```python
from build123d import *

# Parameters (mm, degrees)
F1_DEPTH = 15
F2_R     = 7.5
F3_DEPTH = 105.450168252
F4_R     = 10
F5_DEPTH = 70


with BuildPart() as f1:
    # F0 (on Front) → F1 (new body, symmetric)
    with BuildSketch(Plane.XZ):
        with BuildLine():
            Line((-21.2132034356, -21.2132034356), (-70.7106781187, -70.7106781187))
            ThreePointArc((-70.7106781187, -70.7106781187), (-38.2683432365, -92.3879532511), (0, -100))
            Line((0, -100), (0, -30))
            ThreePointArc((0, -30), (-11.480502971, -27.7163859753), (-21.2132034356, -21.2132034356))
        make_face()
        with BuildLine():
            Line((0, -30), (0, -100))
            ThreePointArc((0, -100), (38.2683432365, -92.3879532511), (70.7106781187, -70.7106781187))
            Line((70.7106781187, -70.7106781187), (21.2132034356, -21.2132034356))
            ThreePointArc((21.2132034356, -21.2132034356), (11.480502971, -27.7163859753), (0, -30))
        make_face()
    extrude(amount=F1_DEPTH, both=True)

    # F2 (on Top) → F3 (cut)
    with BuildSketch(Plane.XY):
        Circle(F2_R)
    extrude(amount=-F3_DEPTH, mode=Mode.SUBTRACT)

    # F4 (on Top) → F5 (cut)
    with BuildSketch(Plane.XY):
        Circle(F4_R)
    extrude(amount=-F5_DEPTH, mode=Mode.SUBTRACT)


solid = f1.part
```
Geometry: final body of the model. Coordinates: model frame, mm. A direction names the side the tool comes from. Coordinates: 2 decimals unless noted, no trailing zeros. Order: outer loops, then holes, each group sorted by start corner. A loop starts at its lowest first (then second) coordinate and runs counter-clockwise, first axis right, second up.
Item 1: Draft query along Y for faces 1 (the face through (46, 0, -46)), 2 (the face through (-1, 15, -60)), 3 (the face through (-7.493, 0.33, -84.79)). Return one class per face: released by +Y, released by -Y, zero draft, split by the parting line, or undercut.
Answer:
face 1: zero draft
face 2: released by +Y
face 3: undercut
Item 2: Material intervals for line 1 along Y through (x, z) = (0, -51); line 2 along X through (y, z) = (6, -25); line 3 along Y through (x, z) = (0, -78), sorted ascending.
Answer:
line 1: y = -15 to -10, 10 to 15
line 2: x = -25 to -16.58, 16.58 to 25
line 3: y = -15 to -7.5, 7.5 to 15
Item 3: Contact query for flat-ended pins moving along their axis: P1, Ø4, axis at y = 0, z = -64.5, coming from the +X side; P2, Ø4, axis at y = 10.5, z = -65.5, coming from the -X side; P3, Ø4, axis at x = -41.5, y = 7, coming from the -Z side. Output: stop coordinate, or through.
Answer:
P1: stops at x = 66.5
P2: stops at x = -67.5
P3: stops at z = -91.87
Item 4: Section query B-B (y = -4). Output: boundary loops of the cut face in (x, z).
Answer:
outline: (-70.71, -70.71) arc R100 ccw to (-6.34, -99.8) - (-6.34, -70) - (-9.17, -70) - (-9.17, -28.57) arc R30 cw to (-21.21, -21.21) - close; (6.34, -99.8) arc R100 ccw to (70.71, -70.71) - (21.21, -21.21) arc R30 cw to (9.17, -28.57) - (9.17, -70) - (6.34, -70) - close
Item 5: Access query for faces 4 (the face through (-2.17, -9.76, -48.85)), 5 (the face through (-1.1, 9.79, -99.994)). Directions: +Z, -Z, +X, -X, +Y, -Y. A direction counts if a zero-diameter tool reaches every point of the face in a straight line with its end or side. Return the directions, or none.
Answer:
face 4: +Z
face 5: -Z, +Y, -Y
Item 6: Section query C-C (z = -52). Output: boundary loops of the cut face in (x, y), then the cut area to 3 significant figures.
Answer:
outline: (-52, -15) - (52, -15) - (52, 15) - (-52, 15) - close; hole circle Ø20 at (0, 0)
area: 2,810 mm2
Item 7: Section query D-D (y = 2). Output: boundary loops of the cut face in (x, z), then the cut area to 3 significant figures.
Answer:
outline: (-70.71, -70.71) arc R100 ccw to (-7.23, -99.74) - (-7.23, -70) - (-9.8, -70) - (-9.8, -28.35) arc R30 cw to (-21.21, -21.21) - close; (7.23, -99.74) arc R100 ccw to (70.71, -70.71) - (21.21, -21.21) arc R30 cw to (9.8, -28.35) - (9.8, -70) - (7.23, -70) - close
area: 5,920 mm2
Item 8: Section query A-A (z = -66.5). Output: boundary loops of the cut face in (x, y).
Answer:
outline: (-66.5, -15) - (66.5, -15) - (66.5, 15) - (-66.5, 15) - close; hole circle Ø20 at (0, 0)
